Autodesk Inventor part; units mm, degrees
ref_plane "YZ Plane" through (0, 0, 0) normal (1, 0, 0) x (0, 1, 0)
ref_plane "XZ Plane" through (0, 0, 0) normal (0, 1, 0) x (-1, 0, 0)
ref_plane "XY Plane" through (0, 0, 0) normal (0, 0, 1) x (1, 0, 0)
sketch "Sketch1" plane through (0, 0, 0) normal (0, 0, 1) x (1, 0, 0)
  circle A0 centre (-3.6979, 7.9302) radius 2.5 construction
  circle A1 centre (3.6979, -7.9302) radius 2.5 construction
  line L0 (-8.2294, 5.8171) -> (-0.8336, -10.0433) construction
  arc A2 (-0.8336, -10.0433) -> (8.2294, -5.8171) centre (3.6979, -7.9302) ccw construction
  line L1 (8.2294, -5.8171) -> (0.8336, 10.0433) construction
  arc A3 (0.8336, 10.0433) -> (-8.2294, 5.8171) centre (-3.6979, 7.9302) ccw construction
  circle A4 centre (78.5293, 90.1574) radius 2.5 construction
  circle A5 centre (94.3897, 82.7616) radius 2.5 construction
  line L2 (76.4162, 85.6259) -> (92.2766, 78.2301) construction
  arc A6 (92.2766, 78.2301) -> (96.5028, 87.2931) centre (94.3897, 82.7616) ccw construction
  line L3 (96.5028, 87.2931) -> (80.6424, 94.689) construction
  arc A7 (80.6424, 94.689) -> (76.4162, 85.6259) centre (78.5293, 90.1574) ccw construction
  circle A8 centre (-75.543, 162.0025) radius 75 construction
  line L4 (112.457, 50.5739) -> (112.457, -27.9975) construction
  line L5 (107.457, -32.9975) -> (39.927, -32.9975) construction
  line L6 (-75.543, 162.0025) -> (58.8073, 27.6522) construction
  line L7 (54.2111, 23.056) -> (63.4035, 32.2484)
  line L8 (70.4745, 32.2484) -> (91.6877, 11.0352)
  line L9 (54.2111, 15.985) -> (75.4243, -5.2282)
  line L10 (75.4243, -12.2993) -> (70.027, -17.6966)
  line L11 (98.7588, 11.0352) -> (104.1561, 16.4325)
  line L12 (-0.8336, -10.0433) -> (-8.2294, 5.8171)
  line L13 (80.6424, 94.689) -> (96.5028, 87.2931)
  arc A9 (-5.811, 12.4617) -> (73.9978, 92.2705) centre (-75.543, 162.0025) ccw
  line L14 (-3.6979, 7.9302) -> (3.6979, -7.9302) construction
  line L15 (78.5293, 90.1574) -> (94.3897, 82.7616) construction
  line L16 (65.9977, -19.1366) -> (3.2042, -12.9058)
  line L17 (105.5961, 20.4618) -> (99.3653, 83.2553)
  arc A10 (75.4243, -12.2993) -> (75.4243, -5.2282) centre (71.8887, -8.7638) ccw
  arc A11 (54.2111, 23.056) -> (54.2111, 15.985) centre (57.7466, 19.5205) ccw
  arc A12 (70.4745, 32.2484) -> (63.4035, 32.2484) centre (66.939, 28.7129) ccw
  arc A13 (91.6877, 11.0352) -> (98.7588, 11.0352) centre (95.2233, 14.5708) ccw
  arc A14 (104.1561, 16.4325) -> (105.5961, 20.4618) centre (100.6206, 19.9681) ccw
  arc A15 (99.3653, 83.2553) -> (96.5028, 87.2931) centre (94.3897, 82.7616) ccw
  arc A16 (80.6424, 94.689) -> (73.9978, 92.2705) centre (78.5293, 90.1574) ccw
  arc A17 (-5.811, 12.4617) -> (-8.2294, 5.8171) centre (-3.6979, 7.9302) ccw
  arc A18 (-0.8336, -10.0433) -> (3.2042, -12.9058) centre (3.6979, -7.9302) ccw
  arc A19 (65.9977, -19.1366) -> (70.027, -17.6966) centre (66.4914, -14.1611) ccw
  point P0 (0, 0)
  point P1 (79.4008, -9.1758)
  point P2 (50.6755, 19.5205)
  point P3 (66.939, 35.784)
  point P4 (95.2233, 7.4997)
  point P5 (78.9598, -8.7638)
  point P6 (68.3532, -19.3704)
  point P7 (105.8299, 18.1063)
  point P8 (0.37, -12.6245)
  point P9 (76.0422, 96.8341)
  point P10 (99.084, 86.0895)
  point P11 (-10.3746, 10.4173)
  point P12 (-4.5315, -2.1131)
  point P13 (88.5726, 90.991)
  dimension "d56" = 190
  dimension "d64" = 23
  dimension "d65" = 40
  dimension "d67" = 165
  dimension "d68" = 15
  dimension "d69" = 15
  dimension "d70" = 20
  dimension "d73" = 5
extrude "Extrusion1" add sketch "Sketch1" along normal blind 5
sketch "Sketch2" plane through (0, 0, 5) normal (0, 0, 1) x (1, 0, 0)
  circle A0 centre (3.6979, -7.9302) radius 2.067
  circle A1 centre (-3.6979, 7.9302) radius 2.067
  circle A2 centre (94.3897, 82.7616) radius 2.067
  circle A3 centre (78.5293, 90.1574) radius 2.067
  point P0 (0, 0)
hole "Hole1" at (78.5293, 90.1574, 5) at (94.3897, 82.7616, 5) at (-3.6979, 7.9302, 5) at (3.6979, -7.9302, 5) direction (0, 0, -1) diameter 5 end through all
sketch "Sketch4" plane through (0, 0, 5) normal (0, 0, 1) x (1, 0, 0)
  circle A0 centre (-3.6979, 7.9302) radius 2.5
  circle A1 centre (78.5293, 90.1574) radius 2.5
  circle A2 centre (94.3897, 82.7616) radius 2.5
  circle A3 centre (3.6979, -7.9302) radius 2.5
  line L0 (-75.543, 162.0025) -> (23.1121, 21.1084) construction
  line L1 (-75.543, 162.0025) -> (-3.6979, 7.9302) construction
  line L2 (78.5293, 90.1574) -> (-75.543, 162.0025) construction
  line L3 (-75.543, 162.0025) -> (65.3511, 63.3474) construction
  circle A4 centre (-75.543, 162.0025) radius 75
  point P0 (0, 0)
  dimension "d27" = 10
  dimension "d28" = 10
  dimension "d71" = 172
  dimension "d72" = 172
hole "Hole2" at (23.1121, 21.1084, 5) at (65.3511, 63.3474, 5) direction (0, 0, -1) diameter 10 end through all
sketch "Sketch6" plane through (0, 0, 5) normal (0, 0, 1) x (1, 0, 0)
  line L0 (23.1121, 21.1084) -> (7.9578, 10.4972) construction
  line L1 (23.1121, 21.1084) -> (38.2664, 31.7195) construction
  line L2 (23.1121, 21.1084) -> (19.0971, 26.8424) construction
  line L3 (65.3511, 63.3474) -> (54.74, 48.1931) construction
  line L4 (65.3511, 63.3474) -> (75.9623, 78.5017) construction
  line L5 (65.3511, 63.3474) -> (59.6171, 67.3624) construction
  arc A0 (-5.811, 12.4617) -> (73.9978, 92.2705) centre (-75.543, 162.0025) ccw
  point P0 (0, 0)
  point P1 (76.0422, 96.8341)
  point P2 (-10.3746, 10.4173)
  dimension "d29" = 18.5
  dimension "d30" = 18.5
  dimension "d38" = 18.5
  dimension "d39" = 18.5
hole "Hole3" at (7.9578, 10.4972, 5) at (38.2664, 31.7195, 5) at (54.74, 48.1931, 5) at (75.9623, 78.5017, 5) direction (0, 0, -1) diameter 4.134 end through all
sketch "Sketch7" plane through (0, 0, 5) normal (0, 0, 1) x (1, 0, 0)
  arc A0 (50.3958, 16.2647) -> (52.016, 14.6445) centre (51.5594, 15.8082) ccw
  arc A1 (56.0526, 10.6079) -> (57.6728, 8.9877) centre (57.2163, 10.1513) ccw
  arc A2 (61.7095, 4.951) -> (63.3297, 3.3308) centre (62.8731, 4.4945) ccw
  arc A3 (67.3663, -0.7058) -> (68.9865, -2.326) centre (68.53, -1.1624) ccw
  arc A4 (71.815, 34.4435) -> (70.1948, 36.0637) centre (70.6513, 34.9001) ccw
  arc A5 (77.4718, 28.7867) -> (75.8516, 30.4069) centre (76.3082, 29.2432) ccw
  arc A6 (83.1287, 23.1298) -> (81.5085, 24.75) centre (81.965, 23.5864) ccw
  arc A7 (88.7855, 17.473) -> (87.1653, 19.0932) centre (87.6219, 17.9295) ccw
  arc A8 (63.5065, 35.8869) -> (61.8863, 34.2668) centre (63.0499, 34.7233) ccw
  arc A9 (52.1927, 24.5732) -> (50.5726, 22.953) centre (51.7362, 23.4096) ccw
  point P0 (0, 0)
hole "Hole4" at (51.7362, 23.4096, 5) at (63.0499, 34.7233, 5) at (51.5594, 15.8082, 5) at (57.2163, 10.1513, 5) at (62.8731, 4.4945, 5) at (70.6513, 34.9001, 5) at (76.3082, 29.2432, 5) at (81.965, 23.5864, 5) at (68.53, -1.1624, 5) at (87.6219, 17.9295, 5) direction (0, 0, -1) diameter 2.5 end through all
properties part number "motorplate"
The model under review builds one solid part; all positions refer to its coordinate system, in mm. A direction names the side the tool comes from. Round coordinates to 2 decimals unless told otherwise and drop trailing zeros. Write each loop counter-clockwise with the first axis right and the second up, starting at its lowest first coordinate (ties: lowest second). Pieces come first, ordered by that corner, then holes.
(1) Wall thickness on L1, parallel to Y at x = 61, z = 4.15; L2, parallel to Y at x = 58, z = 2.1; L3, parallel to Y at x = 68.53, z = 3.15: over which ranges is each line inside the solid? List them lowest first.
(2) Insertion check: pin 1 (1.5 mm diameter, centred on x = 43.5, z = 2, fed in from +Y); pin 2 (3 mm diameter, centred on x = 7, z = 1, fed in from -Y); pin 3 (4.5 mm diameter, centred on x = -3.7, y = 7.93, fed in from -Z); pin 4 (4 mm diameter, centred on x = 57.22, y = 10.15, fed in from +Z). Each pin has a flat end and moves straight along its axis. Give the tip position at first contact, or say it passes through.
(3) Mouldability with a two-part tool opening along Y and no side actions: class faces 1 (the cylindrical face through (98.45, 85.68, 2.46)), 2 (the cylindrical face through (18.155, 21.759, 2.465)), 3 (the flat face through (72.763, -14.96, 2.465)) as +Y half, -Y half, draft (parallel to the pull), parting line (faces both ways), or undercut.
(4) We need section A-A on z = 2.3. Give the number of separate pieces and of enclosed holes in the cut face, and give its area (3 significant figures).
(5) Machinability: for faces 4 (the flat face through (64.669, 5.527, 2.465)), 5 (the flat face through (48, 26, 0)), which of the approach directions +Z, -Z, +X, -X, +Y, -Y give a long, thin tool a straight path to every point of the face, cutting with its end or side? Answer none if there is none.
(6) We need section B-B on y = 53.5. Give the boundary of the cut face in (x, z), and give its area (3 significant figures).
Findings below:
1. L1: y = -18.64 to 9.2, 29.84 to 60.88, 65.81 to 69.37
1. L2: y = -18.34 to 9.18, 11.13 to 12.2, 26.84 to 65.09
1. L3: y = -18.73 to -2.41, 0.09 to 1.67, 33.45 to 59.49, 67.21 to 81.58
2. pin 1: stops at y = 48.54
2. pin 2: stops at y = -13.43
2. pin 3: passes through
2. pin 4: stops at z = 5
3. face 1: +Y half
3. face 2: undercut
3. face 3: -Y half
4. separate pieces: 1
4. enclosed holes: 20
4. area: 5,980 mm2
5. face 4: +Z, -Z
5. face 5: -Z, +X, -X, +Y, -Y
6. outline: (48.76, 0) - (102.32, 0) - (102.32, 5) - (48.76, 5) - close
6. area: 268 mm2
